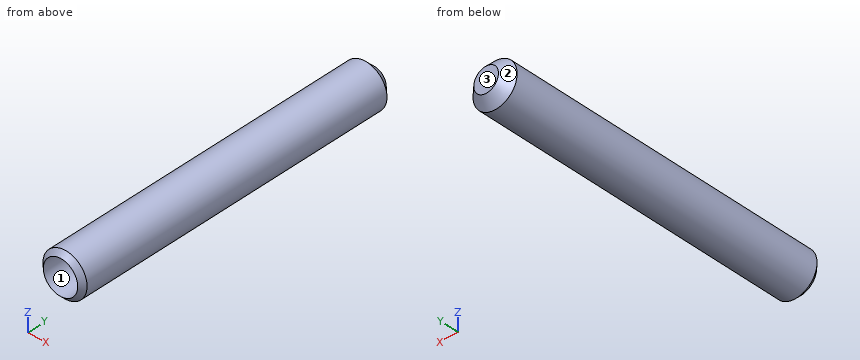
from build123d import *

# Parameters (mm, degrees)
F0_R     = 11.3287531589
F1_DEPTH = 177.1
F2_DEPTH = 52.2
F3_SIZE  = 5
F4_T     = -2.5


with BuildPart() as f1:
    # F0 (on Front) → F1 (new body)
    with BuildSketch(Plane.XZ):
        Circle(F0_R)
    extrude(amount=F1_DEPTH)

    # F2 (add): a face of the model
    f2_faces = [f1.faces().sort_by_distance(p)[0] for p in [
        (0, -177.1, 0),
    ]]
    extrude(f2_faces, amount=-F2_DEPTH)

    # F3
    f3_edges = [f1.edges().sort_by_distance(p)[0] for p in [
        (-11.328753, -177.1, 0),
        (-11.328753, 0, 0),
    ]]
    chamfer(f3_edges, length=F3_SIZE)

    # F4
    f4_openings = [f1.faces().sort_by_distance(p)[0] for p in [
        (0, -177.1, 0),
        (-8.828753, -174.6, 0),
    ]]
    offset(amount=F4_T, openings=f4_openings)


solid = f1.part
Here's how the part is built. I have some questions about the finished solid (model axes, mm). Face numbers are marked on the shaded views. Round coordinates to 2 decimals unless told otherwise and drop trailing zeros. Write each loop counter-clockwise with the first axis right and the second up, starting at its lowest first coordinate (ties: lowest second). Pieces come first, ordered by that corner, then holes.
1. I need wall thicknesses on L1, parallel to Z at x = -0.75, y = -114.5; L2, parallel to X at y = -18, z = 0.25; L3, parallel to Z at x = 2.5, y = -135.5. Which ranges of each line are inside material? Lowest first, please.
2. Will these pins go through, and if not, where does the flat tip stop? pin 1 Ø4 at (x, z) = (8.5, 0.5) entering from +Y; pin 2 Ø6 at (x, y) = (4, -117) entering from +Z; pin 3 Ø4 at (y, z) = (-54, 6) entering from -X.
3. Suppose I cut it at A-A (x = 0). List the corners of the cut face in (y, z) for me, and give its area (3 significant figures).
4. Suppose I cut it at C-C (y = -87). List the corners of the cut face in (x, z) for me, and give its area (3 significant figures).
5. Suppose I cut it at B-B (z = 0). List the corners of the cut face in (x, y) for me.
6. If we mould it in two halves opening along Z, with no side actions, what happens to the marked faces 1, 2 and 3? For each: released by +Z, released by -Z, zero draft, split by the parting line, or undercut.
Answer sheet:
1. L1: z = -11.3 to -8.8, 8.8 to 11.3
1. L2: x = -11.33 to -8.83, 8.83 to 11.33
1. L3: z = -11.05 to -8.47, 8.47 to 11.05
2. pin 1: stops at y = -0.19
2. pin 2: stops at z = 11.28
2. pin 3: stops at x = -10.6
3. outline: (-174.6, -8.83) - (-172.1, -11.33) - (-5, -11.33) - (0, -6.33) - (0, 6.33) - (-5, 11.33) - (-172.1, 11.33) - (-174.6, 8.83) - (-6.04, 8.83) - (-2.5, 5.29) - (-2.5, -5.29) - (-6.04, -8.83) - close
3. area: 898 mm2
4. outline: circle Ø22.66 at (0, 0); hole circle Ø17.66 at (0, 0)
4. area: 158 mm2
5. outline: (-11.33, -172.1) - (-8.83, -174.6) - (-8.83, -6.04) - (-5.29, -2.5) - (5.29, -2.5) - (8.83, -6.04) - (8.83, -174.6) - (11.33, -172.1) - (11.33, -5) - (6.33, 0) - (-6.33, 0) - (-11.33, -5) - close
6. face 1: undercut
6. face 2: split by the parting line
6. face 3: zero draft
